Work out the finished part from the listing and answer in its coordinate system (mm). A direction names the side the tool comes from. Round coordinates to 2 decimals unless told otherwise and drop trailing zeros. Loops run counter-clockwise (first coordinate to the right, second up) from the corner with the lowest first, then second, coordinate; pieces in that order, holes last. Notation, with made-up numbers: (15, -4) - (36, -4) arc R22 ccw to (36, 25) - close; hole circle Ø8 at (38, 80.5). An arc over 180 degrees is marked (long way). Answer as CSV lines item,"result". Start each with the question number.
```python
from build123d import *

# Parameters (mm, degrees)
BOSS_EXTRUDE1_DEPTH = 600
SKETCH4_W           = 112
SKETCH4_H           = 100
BOSS_EXTRUDE2_DEPTH = 8.5
SKETCH6_R           = 3.3
CUT_EXTRUDE1_DEPTH  = 9.5
SKETCH7_R           = 6.5
CUT_EXTRUDE2_DEPTH  = 6.6


with BuildPart() as part:
    # Sketch1 → Boss-Extrude1 (new body)
    with BuildSketch(Plane.XY):
        Polygon((0, 0), (95, 0), (95, 15), (75, 15), (75, 23.5), (103.5, 23.5), (103.5, -8.5), (-8.5, -8.5), (-8.5, 23.5), (20, 23.5), (20, 15), (0, 15), align=None)
    extrude(amount=BOSS_EXTRUDE1_DEPTH)

    # Sketch4 → Boss-Extrude2 (add)
    with BuildSketch(Plane.XZ.offset(8.5)):
        with Locations((47.5, 650)):
            Rectangle(SKETCH4_W, SKETCH4_H)
    extrude(amount=-BOSS_EXTRUDE2_DEPTH)

    # Sketch6 → Cut-Extrude1 (cut, through all)
    with BuildSketch(Plane(origin=(0, 0, 0), x_dir=(1, 0, 0), z_dir=(0, 1, 0))):
        with Locations((47.5, -240)):
            Circle(SKETCH6_R)
        with Locations((47.5, -292)):
            Circle(SKETCH6_R)
        with Locations((47.5, -344)):
            Circle(SKETCH6_R)
        with Locations((47.5, -396)):
            Circle(SKETCH6_R)
    extrude(amount=-CUT_EXTRUDE1_DEPTH, mode=Mode.SUBTRACT)

    # Sketch7 → Cut-Extrude2 (cut)
    with BuildSketch(Plane(origin=(0, 0, 0), x_dir=(1, 0, 0), z_dir=(0, 1, 0))):
        with Locations((47.5, -240)):
            Circle(SKETCH7_R)
        with Locations((47.5, -292)):
            Circle(SKETCH7_R)
        with Locations((47.5, -344)):
            Circle(SKETCH7_R)
        with Locations((47.5, -396)):
            Circle(SKETCH7_R)
    extrude(amount=-CUT_EXTRUDE2_DEPTH, mode=Mode.SUBTRACT)


solid = part.part
```
Item 1: Section D-D, the plane z = 650 is taken. Give the vertices of the cut face in (x, y).
Item 2: Section B-B, the plane z = 43.5 is taken. Give the vertices of the cut face in (x, y), and give its area (3 significant figures).
Item 3: Determine the mould class of faces 4 (the face through (50, -6.6, 399)), 5 (the face through (89, 23.5, 296)), 6 (the face through (50.994, -3.254, 390.519)), 7 (the face through (3, 17, 600)) for opening direction Z: pulls with the +Z half, pulls with the -Z half, needs draft (parallel to the pull), parting line crosses it, or undercut.
Item 4: Section A-A, the plane x = 86 is taken. Give the vertices of the cut face in (y, z), and give its area (4 significant figures).
Item 5: Which of the six approach directions +Z, -Z, +X, -X, +Y, -Y give full straight-line access (tool end or side, diameter ignored) to faces 1 (the face through (46.091, -3.254, 246.345)), 2 (the face through (93, 17, 600)), 3 (the face through (10, 15, 296))?
Item 6: Find the intervals of material crossed by L1, parallel to Z at x = 47, y = -7; L2, parallel to Z at x = 47.5, y = -2.25; L3, parallel to X at y = 16.5, z = 470, in increasing order.
Item 7: Flat-ended cylindrical pins translate along their axes: pin 1 Ø8 at (x, z) = (49, 470.5) entering from +Y; pin 2 Ø6.5 at (x, z) = (49, 241) entering from +Y; pin 3 Ø7 at (x, y) = (6, 14) entering from +Z. Find the tip coordinate at first contact, or state that the pin passes through.
Item 8: Section C-C, the plane x = 34 is taken. Give the vertices of the cut face in (y, z).
Answer:
1,outline,"(-8.5, -8.5) - (103.5, -8.5) - (103.5, 0) - (-8.5, 0) - close"
2,outline,"(-8.5, -8.5) - (103.5, -8.5) - (103.5, 23.5) - (75, 23.5) - (75, 15) - (95, 15) - (95, 0) - (0, 0) - (0, 15) - (20, 15) - (20, 23.5) - (-8.5, 23.5) - close"
2,area,"1,690 mm²"
3,face 4,"undercut"
3,face 5,"needs draft"
3,face 6,"undercut"
3,face 7,"pulls with the +Z half"
4,outline,"(-8.5, 0) - (0, 0) - (0, 700) - (-8.5, 700) - close; (15, 0) - (23.5, 0) - (23.5, 600) - (15, 600) - close"
4,area,"11,050 mm²"
5,face 1,"+Y"
5,face 2,"+Z, +X, -X, +Y"
5,face 3,"+Z, -Z"
6,L1,"z = 0 to 236.74, 243.26 to 288.74, 295.26 to 340.74, 347.26 to 392.74, 399.26 to 700"
6,L2,"z = 0 to 233.5, 246.5 to 285.5, 298.5 to 337.5, 350.5 to 389.5, 402.5 to 700"
6,L3,"x = -8.5 to 20, 75 to 103.5"
7,pin 1,"stops at y = 0"
7,pin 2,"stops at y = -6.6"
7,pin 3,"stops at z = 600"
8,outline,"(-8.5, 0) - (0, 0) - (0, 700) - (-8.5, 700) - close"
